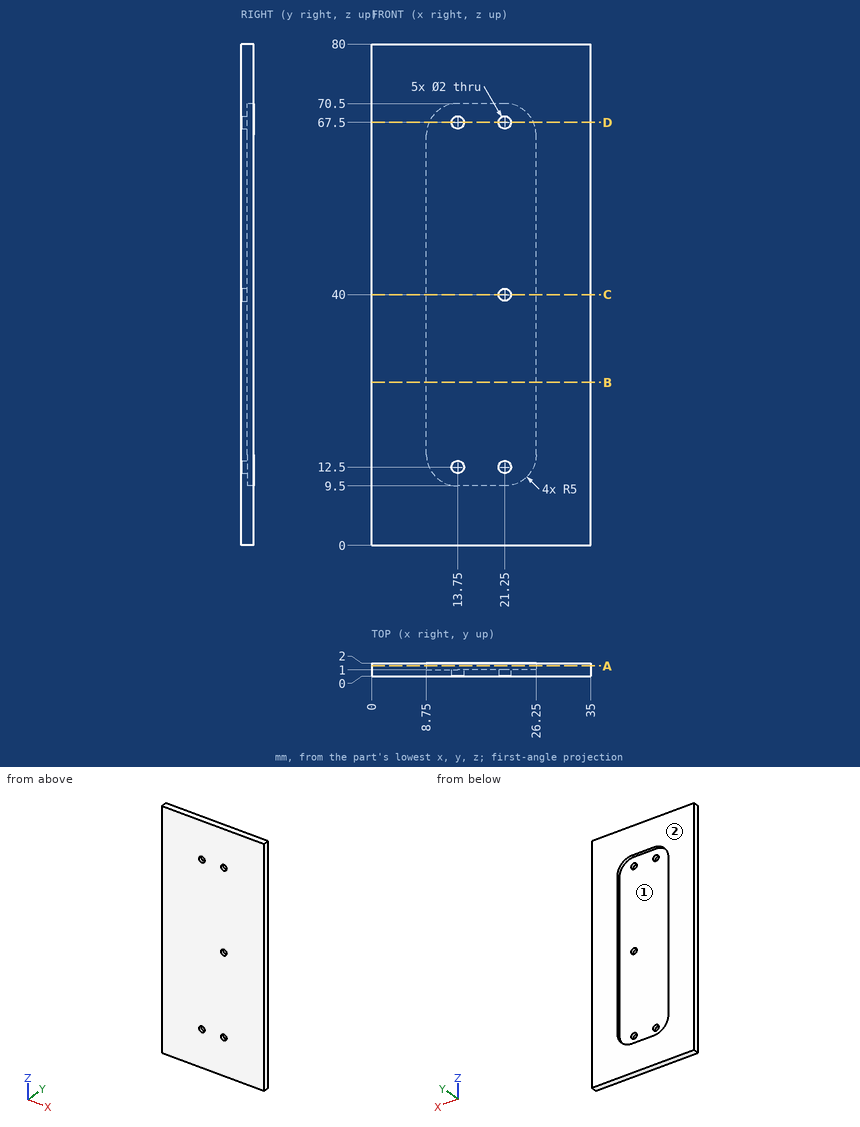
Drawing for the job (mm, zero at the part's lowest x, y, z). Give positions to 0.01 mm unless a question says otherwise; leave off trailing zeros. Loops run counter-clockwise (first coordinate to the right, second up) from the corner with the lowest first, then second, coordinate; pieces in that order, holes last.
(1) Band-saw the part on B-B (z = 26). Write the cut outline in (x, y), and give its area (3 significant figures).
Return value:
outline: (0, 0) - (35, 0) - (35, 2) - (26.25, 2) - (26.25, 1) - (8.75, 1) - (8.75, 2) - (0, 2) - close
area: 52.5 mm2
(2) Pull direction X, two halves, no side cores. Call the marked faces 1 and 2: pulls with the +X half, pulls with the -X half, needs draft (parallel to the pull), parting line crosses it, or undercut.
Return value:
face 1: undercut
face 2: needs draft
(3) Band-saw the part on A-A (y = 1.6). Write the cut outline in (x, z).
Return value:
outline: (0, 0) - (35, 0) - (35, 80) - (0, 80) - close; hole (8.75, 14.5) arc R5 ccw to (13.75, 9.5) - (21.25, 9.5) arc R5 ccw to (26.25, 14.5) - (26.25, 65.5) arc R5 ccw to (21.25, 70.5) - (13.75, 70.5) arc R5 ccw to (8.75, 65.5) - close
(4) Band-saw the part on C-C (z = 40). Write the cut outline in (x, y).
Return value:
outline: (0, 0) - (20.25, 0) - (20.25, 1) - (8.75, 1) - (8.75, 2) - (0, 2) - close; (22.25, 0) - (35, 0) - (35, 2) - (26.25, 2) - (26.25, 1) - (22.25, 1) - close
(5) Drill centre lines: line 1 along Z through (x, y) = (13.75, 0.55); line 2 along X through (y, z) = (1.4, 35); line 3 along Z through (x, y) = (21.25, 0.6). Where is each one in solid material? Low to high.
Return value:
line 1: z = 0 to 11.5, 13.5 to 66.5, 68.5 to 80
line 2: x = 0 to 8.75, 26.25 to 35
line 3: z = 0 to 11.5, 13.5 to 39, 41 to 66.5, 68.5 to 80
(6) Pin check, flat tips, straight feed: pin 1 (2.5 mm diameter, centred on x = 13.75, z = 67.5, fed in from +Y); pin 2 (1.2 mm diameter, centred on x = 13.75, z = 12.5, fed in from +Y); pin 3 (1 mm diameter, centred on x = 29, y = 0.5, fed in from -Z). Stop position of each tip, or through.
Return value:
pin 1: stops at y = 1
pin 2: passes through
pin 3: stops at z = 0
(7) Band-saw the part on D-D (z = 67.5). Write the cut outline in (x, y).
Return value:
outline: (0, 0) - (12.75, 0) - (12.75, 1) - (9.17, 1) - (9.17, 2) - (0, 2) - close; (14.75, 0) - (20.25, 0) - (20.25, 1) - (14.75, 1) - close; (22.25, 0) - (35, 0) - (35, 2) - (25.83, 2) - (25.83, 1) - (22.25, 1) - close
